from build123d import *

# Parameters (mm, degrees)
SKETCH2_R           = 2.4511
BOSS_EXTRUDE1_DEPTH = 12.7


with BuildPart() as part:
    # Sketch2 → Boss-Extrude1 (new body)
    with BuildSketch(Plane(origin=(0, 0, 0), x_dir=(1, 0, 0), z_dir=(0, 1, 0))):
        Polygon((127.583980757, 46.188021535), (127.583980757, -46.188021535), (-23.791990378, -133.584979219), (-103.791990378, -87.396957684), (-103.791990378, 87.396957684), (-23.791990378, 133.584979219), align=None)
        with Locations(Location((69.596393923, -69.745175923, 0), (0, 0, 270))):
            Circle(SKETCH2_R, mode=Mode.SUBTRACT)
        with Locations(Location((25.602897179, -95.144833111, 0), (0, 0, 90))):
            Circle(SKETCH2_R, mode=Mode.SUBTRACT)
        with Locations(Location((60.999643199, -54.855166889, 0), (0, 0, 90))):
            Circle(SKETCH2_R, mode=Mode.SUBTRACT)
        with Locations(Location((17.006146456, -80.254824077, 0), (0, 0, 270))):
            Circle(SKETCH2_R, mode=Mode.SUBTRACT)
        with Locations(Location((-78.005789655, -25.399657187, 0), (0, 0, 90))):
            Circle(SKETCH2_R, mode=Mode.SUBTRACT)
        with Locations(Location((-95.199291102, -25.399657187, 0), (0, 0, 270))):
            Circle(SKETCH2_R, mode=Mode.SUBTRACT)
        with Locations(Location((-95.199291102, 25.399657187, 0), (0, 0, 90))):
            Circle(SKETCH2_R, mode=Mode.SUBTRACT)
        with Locations(Location((-78.005789655, 25.399657187, 0), (0, 0, 270))):
            Circle(SKETCH2_R, mode=Mode.SUBTRACT)
        with Locations(Location((60.999643199, 54.855166889, 0), (0, 0, 270))):
            Circle(SKETCH2_R, mode=Mode.SUBTRACT)
        with Locations(Location((69.596393923, 69.745175923, 0), (0, 0, 90))):
            Circle(SKETCH2_R, mode=Mode.SUBTRACT)
        with Locations(Location((25.602897179, 95.144833111, 0), (0, 0, 270))):
            Circle(SKETCH2_R, mode=Mode.SUBTRACT)
        with Locations(Location((17.006146456, 80.254824077, 0), (0, 0, 90))):
            Circle(SKETCH2_R, mode=Mode.SUBTRACT)
    extrude(amount=BOSS_EXTRUDE1_DEPTH)


solid = part.part
Part model, mm, in its own coordinate system. Coordinates: 2 decimals unless noted, no trailing zeros. Order: outer loops, then holes, each group sorted by start corner. A loop starts at its lowest first (then second) coordinate and runs counter-clockwise, first axis right, second up.
(1) Slice it at C-C, the plane z = 101. Write the cut outline in (x, y), and give its area (3 significant figures).
Check sheet entries:
outline: (-80.23, 0) - (32.65, 0) - (32.65, 12.7) - (-80.23, 12.7) - close
area: 1,430 mm2
(2) Pin check, flat tips, straight feed: pin 1 Ø4.5 at (x, z) = (61, 54.86) entering from -Y; pin 2 Ø2 at (x, y) = (59.5, 2) entering from -Z; pin 3 Ø3 at (x, y) = (96, 4) entering from +Z; pin 4 Ø1 at (x, y) = (16.5, 8) entering from -Z. Stop position of each tip, or through.
Check sheet entries:
pin 1: passes through
pin 2: stops at z = -86.07
pin 3: stops at z = 65.29
pin 4: stops at z = -110.61
(3) Slice it at B-B, the plane x = -46. Write the cut outline in (y, z), and give its area (3 significant figures).
Check sheet entries:
outline: (0, -120.76) - (12.7, -120.76) - (12.7, 120.76) - (0, 120.76) - close
area: 3,070 mm2
(4) Slice it at A-A, the plane y = 8.5. State how many separate pieces and enclosed holes the cut face has, and give its area (3 significant figures).
Check sheet entries:
separate pieces: 1
enclosed holes: 12
area: 44,700 mm2
(5) Probe L1, parallel to X at y = 11, z = 26.5; L2, parallel to Z at x = 59, y = 9.5 (3 decimals); L3, parallel to Z at x = -93, y = 11. List the from-to ranges inside material, lowest first.
Check sheet entries:
L1: x = -103.79 to -97.39, -93.01 to -80.2, -75.82 to 127.58
L2: z = -85.785 to -56.273, -53.438 to 53.438, 56.273 to 85.785
L3: z = -93.63 to -26.48, -24.32 to 24.32, 26.48 to 93.63
